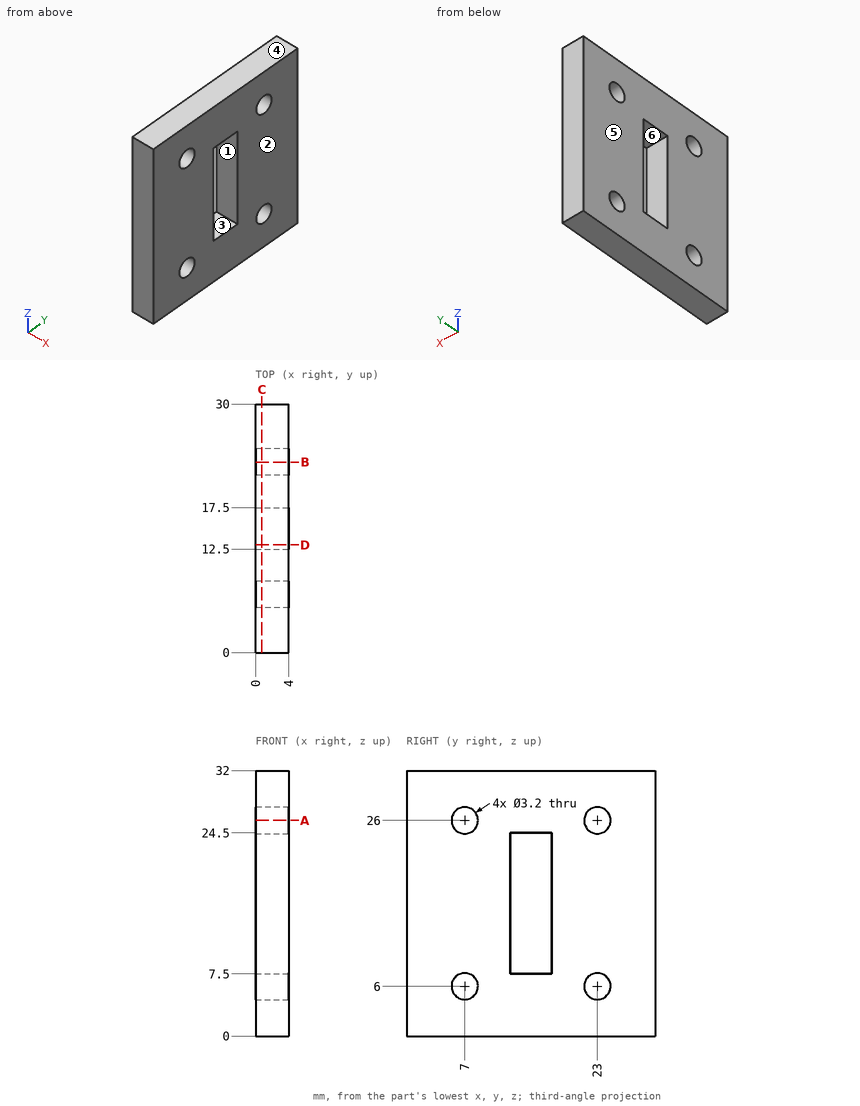
Here's the drawing with two shaded views (mm, measured from the low corner). I have some questions. A direction names the side the tool comes from. Coordinates: 2 decimals unless noted, no trailing zeros. Loops run counter-clockwise (first coordinate to the right, second up) from the corner with the lowest first, then second, coordinate; pieces in that order, holes last. Notation, with made-up numbers: (-16, 50) -> (8, 50) arc R27 ccw to (8, 73) -> close; hole circle Ø2 at (82, 39). An arc over 180 degrees is marked (long way). Answer in a Markdown table with one row per item.
(1) Thinking about a two-plate mould opening in Z: for the marked faces 3, 4, 5 and 6, which applies, released by +Z, released by -Z, zero draft, split by the parting line, or undercut?
Results found:
| item | result |
|---|---|
| face 3 | undercut |
| face 4 | released by +Z |
| face 5 | zero draft |
| face 6 | undercut |
(2) Imagine slicing it at C-C (x = 0.75). List the corners of the cut face in (y, z) for me, plus the area to 3 significant figures.
Results found:
| item | result |
|---|---|
| outline | (0, 0) -> (30, 0) -> (30, 32) -> (0, 32) -> close; hole circle Ø3.2 at (7, 6); hole circle Ø3.2 at (7, 26); hole (12.5, 7.5) -> (17.5, 7.5) -> (17.5, 24.5) -> (12.5, 24.5) -> close; hole circle Ø3.2 at (23, 6); hole circle Ø3.2 at (23, 26) |
| area | 843 mm^2 |
(3) For the marked faces 1 and 2, which set-ups out of +Z, -Z, +X, -X, +Y, -Y let a thin tool reach every point of the face, with its end or its side?
Results found:
| item | result |
|---|---|
| face 1 | +X, -X |
| face 2 | +Z, -Z, +X, +Y, -Y |
(4) Imagine slicing it at A-A (z = 26). List the corners of the cut face in (x, y) for me, plus the area to 3 significant figures.
Results found:
| item | result |
|---|---|
| outline | (0, 0) -> (4, 0) -> (4, 5.4) -> (0, 5.4) -> close; (0, 8.6) -> (4, 8.6) -> (4, 21.4) -> (0, 21.4) -> close; (0, 24.6) -> (4, 24.6) -> (4, 30) -> (0, 30) -> close |
| area | 94.4 mm^2 |
(5) Imagine slicing it at B-B (y = 23). List the corners of the cut face in (x, z) for me.
Results found:
| item | result |
|---|---|
| outline | (0, 0) -> (4, 0) -> (4, 4.4) -> (0, 4.4) -> close; (0, 7.6) -> (4, 7.6) -> (4, 24.4) -> (0, 24.4) -> close; (0, 27.6) -> (4, 27.6) -> (4, 32) -> (0, 32) -> close |
(6) If I drill on probe 1 along Y at (x, z) = (1.3, 6); probe 2 along Y at (x, z) = (2.2, 22); probe 3 along Z at (x, y) = (3.4, 6.5), over which ranges is the centre line in solid material (lowest first)?
Results found:
| item | result |
|---|---|
| probe 1 | y = 0 to 5.4, 8.6 to 21.4, 24.6 to 30 |
| probe 2 | y = 0 to 12.5, 17.5 to 30 |
| probe 3 | z = 0 to 4.48, 7.52 to 24.48, 27.52 to 32 |
(7) Will this pin go through, and if not, where does the flat tip stop? pin 1 Ø2 at (x, z) = (2, 16.5) entering from -Y.
Results found:
| item | result |
|---|---|
| pin 1 | stops at y = 0 |
(8) Imagine slicing it at D-D (y = 13). List the corners of the cut face in (x, z) for me.
Results found:
| item | result |
|---|---|
| outline | (0, 0) -> (4, 0) -> (4, 7.5) -> (0, 7.5) -> close; (0, 24.5) -> (4, 24.5) -> (4, 32) -> (0, 32) -> close |
